from build123d import *

# Parameters (mm, degrees)
ESBO_O1_W                = 7
ESBO_O1_H                = 30
RESSALTO_EXTRUS_O1_DEPTH = 46
RESSALTO_EXTRUS_O2_DEPTH = 11
FILETE1_R                = 3
ESBO_O3_R                = 1.5
CORTE_EXTRUS_O1_DEPTH    = 8
ESBO_O4_W                = 10
ESBO_O4_H                = 46
RESSALTO_EXTRUS_O4_DEPTH = 15
ESBO_O5_R                = 2.75
CORTE_EXTRUS_O2_DEPTH    = 11
ESBO_O6_R                = 4
CORTE_EXTRUS_O3_DEPTH    = 2
ESBO_O7_W                = 7.5
ESBO_O7_H                = 4
RESSALTO_EXTRUS_O5_DEPTH = 11
CORTE_EXTRUS_O4_DEPTH    = 45.25
FILETE2_R                = 3
FILETE3_R                = 3
ESBO_O9_R                = 2
CORTE_EXTRUS_O5_DEPTH    = 22
ESBO_O15_R               = 1.5
CORTE_EXTRUS_O6_DEPTH    = 22
CORTE_EXTRUS_O7_DEPTH    = 2.5


with BuildPart() as part:
    # Esboço1 → Ressalto-extrusão1 (new body)
    with BuildSketch(Plane(origin=(0, 0, 0), x_dir=(1, 0, 0), z_dir=(0, 1, 0))):
        Rectangle(ESBO_O1_W, ESBO_O1_H)
    extrude(amount=RESSALTO_EXTRUS_O1_DEPTH)

    # Esboço2 → Ressalto-extrusão2 (add)
    with BuildSketch(Plane.ZY.offset(3.5)):
        Polygon((0, 40), (-7.5, 40), (-7.5, 29.5), (-15, 29.5), (-15, 46), (15, 46), (15, 29.5), (7.5, 29.5), (7.5, 40), align=None)
    extrude(amount=RESSALTO_EXTRUS_O2_DEPTH)

    # Filete1
    filete1_edges = [part.edges().sort_by_distance(p)[0] for p in [
        (-14.5, 34.75, -7.5),
        (-14.5, 34.75, 7.5),
    ]]
    fillet(filete1_edges, radius=FILETE1_R)

    # Esboço3 → Corte-extrusão1 (cut, through all)
    with BuildSketch(Plane.ZY.offset(3.5)):
        with Locations((-10.25, 5)):
            Circle(ESBO_O3_R)
        with Locations((10.25, 5)):
            Circle(ESBO_O3_R)
        with Locations((-10.25, 22.5)):
            Circle(ESBO_O3_R)
        with Locations((10.25, 22.5)):
            Circle(ESBO_O3_R)
    extrude(amount=-CORTE_EXTRUS_O1_DEPTH, mode=Mode.SUBTRACT)

    # Esboço4 → Ressalto-extrusão4 (add)
    with BuildSketch(Plane(origin=(3.5, 0, 0), x_dir=(0, 0, -1), z_dir=(1, 0, 0))):
        with Locations((10, 23)):
            Rectangle(ESBO_O4_W, ESBO_O4_H)
    extrude(amount=RESSALTO_EXTRUS_O4_DEPTH)

    # Esboço5 → Corte-extrusão2 (cut, through all)
    with BuildSketch(Plane.XY.offset(-5)):
        with Locations((11, 11.5)):
            Circle(ESBO_O5_R)
        with Locations((11, 34.5)):
            Circle(ESBO_O5_R)
    extrude(amount=-CORTE_EXTRUS_O2_DEPTH, mode=Mode.SUBTRACT)

    # Esboço6 → Corte-extrusão3 (cut)
    with BuildSketch(Plane.XY.offset(-5)):
        with Locations((11, 11.5)):
            Circle(ESBO_O6_R)
        with Locations((11, 34.5)):
            Circle(ESBO_O6_R)
    extrude(amount=-CORTE_EXTRUS_O3_DEPTH, mode=Mode.SUBTRACT)

    # Esboço7 → Ressalto-extrusão5 (add)
    with BuildSketch(Plane.XY.offset(-5)):
        with Locations((7.25, 3.75)):
            Rectangle(ESBO_O7_W, ESBO_O7_H)
        with Locations((7.25, 23)):
            Rectangle(ESBO_O7_W, ESBO_O7_H)
        with Locations((7.25, 42.25)):
            Rectangle(ESBO_O7_W, ESBO_O7_H)
    extrude(amount=RESSALTO_EXTRUS_O5_DEPTH)

    # Esboço8 → Corte-extrusão4 (cut, through all)
    with BuildSketch(Plane.XZ.offset(-1.75)):
        Polygon((11, -5), (3.5, 6), (11, 6), align=None)
    extrude(amount=-CORTE_EXTRUS_O4_DEPTH, mode=Mode.SUBTRACT)

    # Filete2
    filete2_edges = [part.edges().sort_by_distance(p)[0] for p in [
        (-5.5, 46, 15),
        (0, 0, 15),
    ]]
    fillet(filete2_edges, radius=FILETE2_R)

    # Filete3
    filete3_edges = [part.edges().sort_by_distance(p)[0] for p in [
        (18.5, 46, -10),
        (18.5, 0, -10),
    ]]
    fillet(filete3_edges, radius=FILETE3_R)

    # Esboço9 → Corte-extrusão5 (cut)
    with BuildSketch(Plane(origin=(0, 0, -15), x_dir=(-1, 0, 0), z_dir=(0, 0, -1))):
        with Locations((11.5, 43)):
            Circle(ESBO_O9_R)
    extrude(amount=-CORTE_EXTRUS_O5_DEPTH, mode=Mode.SUBTRACT)

    # Esboço15 → Corte-extrusão6 (cut)
    with BuildSketch(Plane(origin=(-14.75, 0, -14.75), x_dir=(0, -1, 0), z_dir=(-0.707106781, 0, -0.707106781))):
        with Locations((-38, -6.01040764)):
            Circle(ESBO_O15_R)
    extrude(amount=-CORTE_EXTRUS_O6_DEPTH, mode=Mode.SUBTRACT)

    # Esboço16 → Corte-extrusão7 (cut)
    with BuildSketch(Plane(origin=(0, 0, -15), x_dir=(-1, 0, 0), z_dir=(0, 0, -1))):
        Polygon((6.5, 39.5), (9.5, 43), (11.5, 41), (8.621320344, 38), align=None)
    extrude(amount=-CORTE_EXTRUS_O7_DEPTH, mode=Mode.SUBTRACT)


solid = part.part
Here's how the part is built. I have some questions about the finished solid (model axes, mm). A direction names the side the tool comes from. Give positions to 0.01 mm unless a question says otherwise; leave off trailing zeros. Loops run counter-clockwise (first coordinate to the right, second up) from the corner with the lowest first, then second, coordinate; pieces in that order, holes last. Notation, with made-up numbers: (27.5, 13.5) -> (78.5, 13.5) arc R18 cw to (78.5, 48.5) -> close; hole circle Ø3 at (1, 57). An arc over 180 degrees is marked (long way). One line per item, written item: value.
Q1. Suppose I cut it at C-C on z = -1.5. Please give me the cut outline in (x, y), then the cut area to 3 significant figures.
Answers follow:
outline: (-14.5, 40) -> (-3.5, 40) -> (-3.5, 0) -> (3.5, 0) -> (3.5, 1.75) -> (8.61, 1.75) -> (8.61, 5.75) -> (3.5, 5.75) -> (3.5, 21) -> (8.61, 21) -> (8.61, 25) -> (3.5, 25) -> (3.5, 40.25) -> (8.61, 40.25) -> (8.61, 44.25) -> (3.5, 44.25) -> (3.5, 46) -> (-14.5, 46) -> close; hole circle Ø4 at (-11.5, 43)
area: 437 mm^2
Q2. I'm going to push flat-ended pins straight in: pin 1 Ø12 at (x, y) = (11.5, 22) entering from +Z; pin 2 Ø4 at (x, z) = (6, -0.5) entering from +Y; pin 3 Ø0.9 at (y, z) = (23, -10) entering from -X; pin 4 Ø5 at (x, y) = (11, 11.5) entering from +Z. Where does each tip first touch, or does it pass through?
Answers follow:
pin 1: z = 3.07
pin 2: y = 44.25
pin 3: x = 3.5
pin 4: through
Q3. If I drill on line 1 along Y through (x, z) = (7.5, -2.5); line 2 along Y through (x, z) = (1.5, -10.25); line 3 along X through (y, z) = (43, -8), over which ranges is the centre line in solid material (lowest first)?
Answers follow:
line 1: 1.75 to 5.75, 21 to 25, 40.25 to 44.25
line 2: 0 to 3.5, 6.5 to 21, 24 to 46
line 3: -14.5 to -13.5, -9.5 to 18.5
Q4. On a 3-axis mill with a long thin cutter (end or side, diameter ignored), from which of +Z, -Z, +X, -X, +Y, -Y can I reach the whole of each face in a straight line? I mean faces 1 (the face through (-0.05, 5.07, -11.75)), 2 (the face through (6, 40.25, -1)), 3 (the face through (-9, 29.5, -11)). Say none if no direction works.
Answers follow:
face 1: -X
face 2: +Z, +X
face 3: +Z, -Z, -X, -Y
Q5. Suppose I cut it at B-B on x = 12. Please give me the cut outline in (y, z).
Answers follow:
outline: (0, -15) -> (8.94, -15) -> (8.94, -7) -> (7.63, -7) -> (7.63, -5) -> (0, -5) -> close; (14.06, -15) -> (31.94, -15) -> (31.94, -7) -> (30.63, -7) -> (30.63, -5) -> (15.37, -5) -> (15.37, -7) -> (14.06, -7) -> close; (37.06, -15) -> (46, -15) -> (46, -5) -> (38.37, -5) -> (38.37, -7) -> (37.06, -7) -> close
Q6. Suppose I cut it at D-D on y = 12.5. Please give me the cut outline in (x, z), then the cut area to 3 significant figures.
Answers follow:
outline: (-3.5, -15) -> (8.44, -15) -> (8.44, -7) -> (7.13, -7) -> (7.13, -5) -> (3.5, -5) -> (3.5, 15) -> (-3.5, 15) -> close; (13.56, -15) -> (18.5, -15) -> (18.5, -5) -> (14.87, -5) -> (14.87, -7) -> (13.56, -7) -> close
area: 304 mm^2
Q7. Suppose I cut it at A-A on y = 22.5. Please give me the cut outline in (x, z).
Answers follow:
outline: (-3.5, -15) -> (18.5, -15) -> (18.5, -5) -> (11, -5) -> (3.5, 6) -> (3.5, 8.75) -> (-3.5, 8.75) -> (-3.5, -8.75) -> (3.5, -8.75) -> (3.5, -11.75) -> (-3.5, -11.75) -> close; (-3.5, 11.75) -> (3.5, 11.75) -> (3.5, 15) -> (-3.5, 15) -> close
Q8. We'd pull the mould along Z, two halves only. Please class faces 4 (the face through (-9, 40, 0)), 5 (the face through (3.5, 5, -10)), 6 (the face through (-11, 43, 7)), 7 (the face through (6, 44.25, -1)): pulls with the +Z half, pulls with the -Z half, needs draft (parallel to the pull), parting line crosses it, or undercut.
Answers follow:
face 4: undercut
face 5: undercut
face 6: pulls with the -Z half
face 7: needs draft
